Part print with two shaded views. Sizes in mm from the minimum x, y, z corner. Coordinates: 2 decimals unless noted, no trailing zeros. Write each loop counter-clockwise with the first axis right and the second up, starting at its lowest first coordinate (ties: lowest second). Pieces come first, ordered by that corner, then holes.
Q1. Pull direction X, two halves, no side cores. Call the marked faces 1, 2 and 3: released by +X, released by -X, zero draft, split by the parting line, or undercut.
Q2. Band-saw the part on D-D, the plane x = 24. Write the cut outline in (y, z).
Q3. Band-saw the part on B-B, the plane x = 2.8. Write the cut outline in (y, z), plus the area to 3 significant figures.
Q4. Drill centre lines: probe 1 along X at (y, z) = (2.75, 6.25); probe 2 along X at (y, z) = (3.75, 1); probe 3 along Y at (x, z) = (2.8, 4.75). Where is each one in solid material? Low to high.
Q5. Pin check, flat tip, straight feed: P1, Ø3, axis at x = 2.8, y = 2.75, coming from the -Z side. Stop position of the tip, or through.
Q6. Band-saw the part on A-A, the plane z = 7.5. Write the cut outline in (x, y), plus the area to 3 significant figures.
Q7. Band-saw the part on C-C, the plane y = 2.75. Write the cut outline in (x, z), plus the area to 3 significant figures.
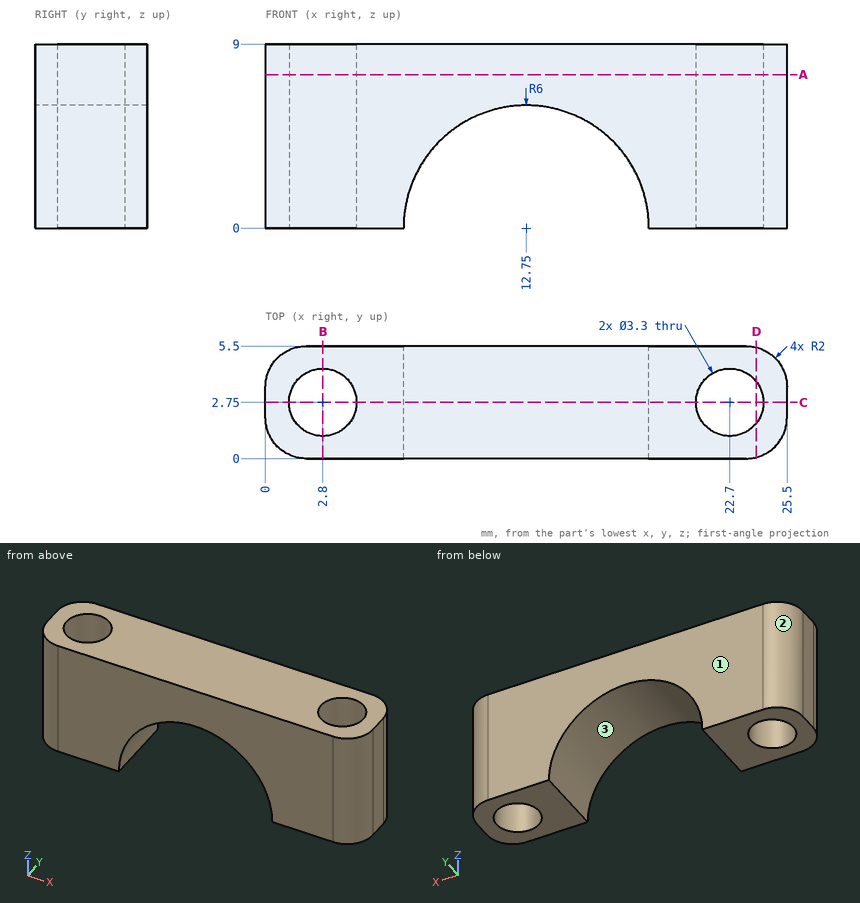
Answer sheet:
1. face 1: zero draft
1. face 2: released by -X
1. face 3: undercut
2. outline: (0.06, 0) - (1.73, 0) - (1.73, 9) - (0.06, 9) - close; (3.77, 0) - (5.44, 0) - (5.44, 9) - (3.77, 9) - close
3. outline: (0, 0) - (1.1, 0) - (1.1, 9) - (0, 9) - close; (4.4, 0) - (5.5, 0) - (5.5, 9) - (4.4, 9) - close
3. area: 19.8 mm2
4. probe 1: x = 0 to 1.15, 4.45 to 21.05, 24.35 to 25.5
4. probe 2: x = 0.02 to 1.49, 4.11 to 6.83, 18.67 to 21.39, 24.01 to 25.48
4. probe 3: y = 0 to 1.1, 4.4 to 5.5
5. P1: passes through
6. outline: (0, 2) arc R2 ccw to (2, 0) - (23.5, 0) arc R2 ccw to (25.5, 2) - (25.5, 3.5) arc R2 ccw to (23.5, 5.5) - (2, 5.5) arc R2 ccw to (0, 3.5) - close; hole circle Ø3.3 at (2.8, 2.75); hole circle Ø3.3 at (22.7, 2.75)
6. area: 120 mm2
7. outline: (0, 0) - (1.15, 0) - (1.15, 9) - (0, 9) - close; (4.45, 0) - (6.75, 0) arc R6 cw to (18.75, 0) - (21.05, 0) - (21.05, 9) - (4.45, 9) - close; (24.35, 0) - (25.5, 0) - (25.5, 9) - (24.35, 9) - close
7. area: 114 mm2
